The listing builds one solid part. Answer for the finished solid, in the listing's coordinates (mm). Face numbers are marked on the shaded views. A direction names the side the tool comes from. Coordinates: 2 decimals unless noted, no trailing zeros. Order: outer loops, then holes, each group sorted by start corner. A loop starts at its lowest first (then second) coordinate and runs counter-clockwise, first axis right, second up. Notation, with made-up numbers: (83, 28.25) - (141, 28.25) arc R22 ccw to (141, 40.25) - close; hole circle Ø3 at (43, 39). An arc over 180 degrees is marked (long way). Use one line per item in the form item = value. Start each with the question number.
Item 1: Section C-C, the plane y = 7.5 is taken. Write down the section's boundary in (x, z).
Item 2: The mould has two halves that part along Z. Classify the marked faces 1, 2 and 3: released by +Z, released by -Z, zero draft, split by the parting line, or undercut.
Item 3: Each of these flat-tipped pins is pushed along its axis until it touches: pin 1 Ø2 at (x, z) = (-1.5, 0.5) entering from +Y; pin 2 Ø4 at (x, z) = (3, -4) entering from -Y (3 decimals); pin 3 Ø2 at (x, y) = (-4.5, 17) entering from -Z. Where does it stop, or does it pass through?
Item 4: Section B-B, the plane z = 0 is taken. Write down the section's boundary in (x, y) (3 decimals).
Item 5: Consider line 1 along Z through (x, y) = (0, 23); line 2 along Z through (x, y) = (0, 7.25); line 3 along Y through (x, z) = (1.5, -5.75). Determine where each line is inside the solid, lowest interval first. Write a range as [from, to].
Item 6: Section D-D, the plane y = 18 is taken. Write down the section's boundary in (x, z).
Item 7: Section A-A, the plane x = 0 is taken. Write down the section's boundary in (y, z) (3 decimals).
Item 8: A tool of negligible diameter and unlimited length cuts with its end or side. For the marked faces 4 and 5, from which of +Z, -Z, +X, -X, +Y, -Y can it reach the whole face along a straight path? Write none if from no direction.
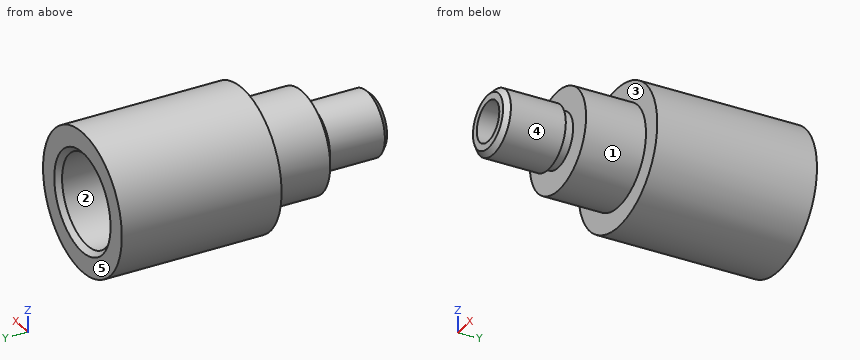
Autodesk Inventor part; units mm, degrees
ref_plane "YZ Plane" through (0, 0, 0) normal (1, 0, 0) x (0, 1, 0)
ref_plane "XZ Plane" through (0, 0, 0) normal (0, 1, 0) x (-1, 0, 0)
ref_plane "XY Plane" through (0, 0, 0) normal (0, 0, 1) x (1, 0, 0)
sketch "Skizze1" plane through (0, 0, 0) normal (0, 0, 1) x (1, 0, 0)
  line L0 (0, 34.8) -> (0, -5.8)
  line L1 (-1.4, 0) -> (8.4, 0)
  line L2 (2, 0) -> (2, 16)
  line L3 (2, 16) -> (4.5, 16)
  line L4 (4.5, 16) -> (4.5, 29)
  line L5 (4.5, 29) -> (7, 29)
  line L6 (7, 29) -> (7, 13)
  line L7 (3.175, 6) -> (3.175, 0)
  line L8 (2, 0) -> (3.175, 0)
  line L9 (5, 7) -> (2.7, 7)
  line L10 (2.7, 7) -> (2.7, 6)
  line L11 (2.7, 6) -> (3.175, 6)
  line L12 (7, 13) -> (5, 13)
  line L13 (5, 13) -> (5, 7)
  point P0 (0, 0)
  dimension "d1" = 1
  dimension "d2" = 2.7
  dimension "d3" = 3.175
  dimension "d4" = 2
  dimension "d5" = 4.5
  dimension "d6" = 13
  dimension "d7" = 7
  dimension "d8" = 5
  dimension "d9" = 6
  dimension "d10" = 3
  dimension "d11" = 7
revolve "Umdrehung1" add sketch "Skizze1" angle 360 about axis through (0, 0, 0) along (0, -1, 0)
chamfer "Fase1" distance 0.5 angle 45 2 edges at (-3.175, 0, 0) (-4.5, 29, 0)
thread "Gewinde1"
thread "Gewinde2"
properties part number "Gewindeadapter" material "Aluminum-6061"
Response:
q1.outline = circle Ø10 at (0, 0); hole circle Ø4 at (0, 0)
q2.face_1 = split by the parting line
q2.face_2 = undercut
q2.face_3 = zero draft
q3.pin_1 = 16
q3.pin_2 = 0.325
q3.pin_3 = -6.06
q4.outline = (-7, 13) - (-5, 13) - (-5, 7) - (-2.7, 7) - (-2.7, 6) - (-3.175, 6) - (-3.175, 0.5) - (-2.675, 0) - (-2, 0) - (-2, 16) - (-4.5, 16) - (-4.5, 28.5) - (-5, 29) - (-7, 29) - close; (2, 0) - (2.675, 0) - (3.175, 0.5) - (3.175, 6) - (2.7, 6) - (2.7, 7) - (5, 7) - (5, 13) - (7, 13) - (7, 29) - (5, 29) - (4.5, 28.5) - (4.5, 16) - (2, 16) - close
q5.line_1 = [-7, -4.5], [4.5, 7]
q5.line_2 = [-5, -2], [2, 5]
q5.line_3 = [13, 29]
q6.outline = circle Ø14 at (0, 0); hole circle Ø9 at (0, 0)
q7.outline = (0, -2.675) - (0.5, -3.175) - (6, -3.175) - (6, -2.7) - (7, -2.7) - (7, -5) - (13, -5) - (13, -7) - (29, -7) - (29, -5) - (28.5, -4.5) - (16, -4.5) - (16, -2) - (0, -2) - close; (0, 2) - (16, 2) - (16, 4.5) - (28.5, 4.5) - (29, 5) - (29, 7) - (13, 7) - (13, 5) - (7, 5) - (7, 2.7) - (6, 2.7) - (6, 3.175) - (0.5, 3.175) - (0, 2.675) - close
q8.face_4 = -Y
q8.face_5 = +Z, -Z, +X, -X, +Y
